from build123d import *

# Parameters (mm, degrees)
BOSS_EXTRUDE1_DEPTH                             = 10
SKETCH2_R                                       = 10
BOSS_EXTRUDE2_DEPTH                             = 15
CUT_EXTRUDE1_START                              = -15
SKETCH2_2_R                                     = 10
CUT_EXTRUDE1_DEPTH                              = 45
CUT_EXTRUDE1_DRAFT                              = 3
CSK_FOR_M6_FLAT_HEAD_MACHINE_SCREW1_D           = 6.6
CSK_FOR_M6_FLAT_HEAD_MACHINE_SCREW1_CSINK_D     = 12.6
CSK_FOR_M6_FLAT_HEAD_MACHINE_SCREW1_CSINK_ANGLE = 90
MIRROR1_START                                   = -15
MIRROR1_COPY_1_SKETCH_R                         = 10
MIRROR1_COPY_1_DEPTH                            = 45
MIRROR1_COPY_1_DRAFT                            = 3
FILLET1_R                                       = 3


with BuildPart() as part:
    # Sketch1 → Boss-Extrude1 (new, symmetric)
    with BuildSketch(Plane.XY):
        with BuildLine():
            Line((-45.5, 0), (-31.87, 0))
            ThreePointArc((-31.87, 0), (0, 31.87), (31.87, 0))
            Line((31.87, 0), (45.5, 0))
            ThreePointArc((45.5, 0), (0, 45.5), (-45.5, 0))
        make_face()
    extrude(amount=BOSS_EXTRUDE1_DEPTH, both=True)

    # Sketch2 → Boss-Extrude2 (add)
    with BuildSketch(Plane.XZ):
        with Locations((-45.5, 0)):
            Circle(SKETCH2_R)
    boss_extrude2 = extrude(amount=-BOSS_EXTRUDE2_DEPTH)


with BuildPart() as cut_extrude1_tool:
    # Sketch2<2> → Cut-Extrude1 (with draft: the straight prism first)
    with BuildSketch(Plane.XZ.offset(CUT_EXTRUDE1_START)):
        with Locations((-45.5, 0)):
            Circle(SKETCH2_2_R)
    extrude(amount=-CUT_EXTRUDE1_DEPTH)
    # Cut-Extrude1: the draft: its side faces are tilted about the plane it starts from
    cut_extrude1_sides = [cut_extrude1_tool.faces().sort_by_distance(p)[0] for p in [
        (-55.5, 37.5, 0),
    ]]
    draft(cut_extrude1_sides, Plane.XZ.offset(CUT_EXTRUDE1_START), CUT_EXTRUDE1_DRAFT)


with BuildPart() as part_1:
    add(part.part)

    # Cut-Extrude1: cut by cut_extrude1_tool
    add(cut_extrude1_tool.part, mode=Mode.SUBTRACT)

    # CSK for M6 Flat Head Machine Screw1 (through all)
    with Locations(Plane(origin=(0, 15, 0), x_dir=(1, 0, 0), z_dir=(0, 1, 0))):
        with Locations((-45.5, 0)):
            csk_for_m6_flat_head_machine_screw1 = CounterSinkHole(CSK_FOR_M6_FLAT_HEAD_MACHINE_SCREW1_D / 2, CSK_FOR_M6_FLAT_HEAD_MACHINE_SCREW1_CSINK_D / 2, counter_sink_angle=CSK_FOR_M6_FLAT_HEAD_MACHINE_SCREW1_CSINK_ANGLE)

    # Mirror1: Boss-Extrude2, CSK for M6 Flat Head Machine Screw1 across plane
    add(boss_extrude2.mirror(Plane(origin=(0, 0, 0), x_dir=(0, 0, 1), z_dir=(1, 0, 0))))
    add(csk_for_m6_flat_head_machine_screw1.mirror(Plane(origin=(0, 0, 0), x_dir=(0, 0, 1), z_dir=(1, 0, 0))), mode=Mode.SUBTRACT)


with BuildPart() as mirror1_copy_1_tool:
    # Mirror1 copy 1 sketch → Mirror1 copy 1 (with draft: the straight prism first)
    with BuildSketch(Plane(origin=(0, 0, 0), x_dir=(-1, 0, 0), z_dir=(0, -1, 0)).offset(MIRROR1_START)):
        with Locations((-45.5, 0)):
            Circle(MIRROR1_COPY_1_SKETCH_R)
    extrude(amount=-MIRROR1_COPY_1_DEPTH)
    # Mirror1 copy 1: the draft: its side faces are tilted about the plane it starts from
    mirror1_copy_1_sides = [mirror1_copy_1_tool.faces().sort_by_distance(p)[0] for p in [
        (55.5, 37.5, 0),
    ]]
    draft(mirror1_copy_1_sides, Plane(origin=(0, 0, 0), x_dir=(-1, 0, 0), z_dir=(0, -1, 0)).offset(MIRROR1_START), MIRROR1_COPY_1_DRAFT)


with BuildPart() as part_2:
    add(part_1.part)

    # Mirror1 copy 1: cut by mirror1_copy_1_tool
    add(mirror1_copy_1_tool.part, mode=Mode.SUBTRACT)

    # Fillet1
    # the kernel refuses this fillet: 3 mm, written as the material it takes off along each edge
    with BuildSketch(Plane(origin=(0, 0, 10), x_dir=(0.9864018839376206, -0.1643512195400838, 0), z_dir=(-0.1643512195400838, -0.9864018839376206, 0))) as fillet1_piece_1_section:
        with BuildLine():
            CenterArc((45.5 - FILLET1_R, -FILLET1_R), FILLET1_R, 0, 90)
            Line((45.5 - FILLET1_R, 0), (45.5, 0))
            Line((45.5, 0), (45.5, -FILLET1_R))
        make_face()
    fillet1_piece_1 = revolve(axis=Axis((0, 0, 10), (0, 0, 1)), revolution_arc=198.919095152, mode=Mode.PRIVATE)
    fillet1_piece_1 = fillet1_piece_1 - Plane(origin=(-45.5, 9.787690876, 0), x_dir=(1, 0, 0), z_dir=(0, -1, 0)) * Cylinder(10, 182, mode=Mode.PRIVATE)
    fillet1_piece_1 = fillet1_piece_1 - Plane(origin=(45.5, 9.787690876, 0), x_dir=(-1, 0, 0), z_dir=(0, -1, 0)) * Cylinder(10, 182, mode=Mode.PRIVATE)
    add(fillet1_piece_1, mode=Mode.SUBTRACT)
    with BuildSketch(Plane(origin=(0, 0, -10), x_dir=(0.9864018839376206, -0.1643512195400838, 0), z_dir=(-0.1643512195400838, -0.9864018839376206, 0))) as fillet1_piece_2_section:
        with BuildLine():
            CenterArc((45.5 - FILLET1_R, FILLET1_R), FILLET1_R, 270, 90)
            Line((45.5 - FILLET1_R, 0), (45.5, 0))
            Line((45.5, 0), (45.5, FILLET1_R))
        make_face()
    fillet1_piece_2 = revolve(axis=Axis((0, 0, -10), (0, 0, 1)), revolution_arc=198.919095152, mode=Mode.PRIVATE)
    fillet1_piece_2 = fillet1_piece_2 - Plane(origin=(-45.5, 9.787689661, 0), x_dir=(1, 0, 0), z_dir=(0, -1, 0)) * Cylinder(10, 182, mode=Mode.PRIVATE)
    fillet1_piece_2 = fillet1_piece_2 - Plane(origin=(45.5, 9.787689661, 0), x_dir=(-1, 0, 0), z_dir=(0, -1, 0)) * Cylinder(10, 182, mode=Mode.PRIVATE)
    add(fillet1_piece_2, mode=Mode.SUBTRACT)


solid = part_2.part
Check sheet for the modelled part. Datum: model origin and axes. Units: mm. A direction names the side the tool comes from. Round coordinates to 2 decimals unless told otherwise and drop trailing zeros. Order: outer loops, then holes, each group sorted by start corner. A loop starts at its lowest first (then second) coordinate and runs counter-clockwise, first axis right, second up.
Q1. Set-up check for faces 1 (the face through (-46, 15, -7)), 2 (the face through (41, 0, 0)), 3 (the face through (46, 15, -7)): record each of +Z, -Z, +X, -X, +Y, -Y from which the full face is reachable in a straight line by a thin tool's end or side.
Filled sheet:
face 1: -X, +Y
face 2: +Z, -Z, +X, -X, -Y
face 3: +X, +Y
Q2. Cross-section at C-C, the plane y = 6.5. Give the number of separate pieces and of enclosed holes in the cut face, plus the area to 3 significant figures.
Filled sheet:
separate pieces: 2
enclosed holes: 2
area: 817 mm2
Q3. Scan lines: L1, parallel to Z at x = -45.5, y = 5.25; L2, parallel to Y at x = 0, z = -4.25; L3, parallel to Y at x = 51, z = -6. Record each from-to range of solid material in increasing order.
Filled sheet:
L1: z = -10 to -3.3, 3.3 to 10
L2: y = 31.87 to 45.5
L3: y = 0 to 15
Q4. Cross-section at A-A, the plane z = 0. Enter the section's corners in (x, y), plus the area to 3 significant figures.
Filled sheet:
outline: (-55.5, 0) - (-48.8, 0) - (-48.8, 12) - (-51.8, 15) - (-55.5, 15) - close; (-42.2, 0) - (-31.87, 0) arc R31.87 cw to (31.87, 0) - (42.2, 0) - (42.2, 12) - (39.2, 15) - (35.5, 15) - (34.75, 29.38) arc R45.5 ccw to (-34.75, 29.38) - (-35.5, 15) - (-39.2, 15) - (-42.2, 12) - close; (48.8, 0) - (55.5, 0) - (55.5, 15) - (51.8, 15) - (48.8, 12) - close
area: 1,640 mm2
Q5. Draft check along Z on faces 4 (the face through (-1, 36, 10)), 5 (the face through (-41, 0, 0)), 6 (the face through (-35.214, 20.49, -0.172)). Enter one of: pulls with the +Z half, pulls with the -Z half, needs draft (parallel to the pull), parting line crosses it, or undercut.
Filled sheet:
face 4: pulls with the +Z half
face 5: needs draft
face 6: undercut
Q6. Depth check by flat-ended pin: P1, Ø4, axis at y = 7, z = 1.5, coming from the +X side; P2, Ø1, axis at y = 6, z = 1, coming from the -X side; P3, Ø7.5, axis at x = -45.5, z = 0, coming from the +Y side; P4, Ø1, axis at x = 26, z = -1.5, coming from the +Y side. Enter the tip coordinate at first touch or a pass-through.
Filled sheet:
P1: stops at x = 55.5
P2: stops at x = -55.49
P3: stops at y = 12.45
P4: stops at y = 37.68
Q7. Cross-section at B-B, the plane x = 0. Enter the section's corners in (y, z).
Filled sheet:
outline: (31.87, -10) - (42.5, -10) arc R3 ccw to (45.5, -7) - (45.5, 7) arc R3 ccw to (42.5, 10) - (31.87, 10) - close
